```python
from build123d import *

# Parameters (mm, degrees)
F0_R     = 60
F1_DEPTH = 75
F2_R     = 45.05
F3_DEPTH = 300
F4_W     = 23.5
F4_H     = 7.8
F5_DEPTH = 78.9


with BuildPart() as f1:
    # F0 (on Front) → F1 (new body, symmetric)
    with BuildSketch(Plane.XZ):
        Circle(F0_R)
    extrude(amount=F1_DEPTH, both=True)

    # F2 (on face) → F3 (cut)
    with BuildSketch(Plane.XZ.offset(75)):
        Circle(F2_R)
    extrude(amount=-F3_DEPTH, mode=Mode.SUBTRACT)

    # F4 (on Right) → F5 (cut, symmetric)
    with BuildSketch(Plane.YZ):
        Rectangle(F4_W, F4_H)
    extrude(amount=F5_DEPTH, both=True, mode=Mode.SUBTRACT)


solid = f1.part
```
Geometry check sheet. Reference: the model listing, model coordinates, mm. A direction names the side the tool comes from. Round coordinates to 2 decimals unless told otherwise and drop trailing zeros. Order: outer loops, then holes, each group sorted by start corner. A loop starts at its lowest first (then second) coordinate and runs counter-clockwise, first axis right, second up. Notation, with made-up numbers: M 60.5,-23.75 L 79.5,-23.75 A23 ccw 79.5,-8.75 Z; hole C 69.5,78 d2. An arc over 180 degrees is marked long. Answer as CSV lines item,"result".
1) Gauge pin test, flat ends, axial feed: pin 1 Ø4.5 at (x, y) = (-49.5, 0) entering from +Z; pin 2 Ø7.5 at (x, y) = (52, -1) entering from -Z; pin 3 Ø12 at (x, y) = (-1, -22.5) entering from +Z. Record the tip position at first contact, or that the pin passes through.
Entries:
pin 1,"z = 36.98"
pin 2,"z = -35.66"
pin 3,"z = 60"
2) Sectioned sample at C-C on x = 0. Record the cut outline in (y, z).
Entries:
outline,"M -75,-60 L 75,-60 L 75,-45.05 L -75,-45.05 Z; M -75,45.05 L 75,45.05 L 75,60 L -75,60 Z"
3) Sectioned sample at D-D on y = -23. Record the cut outline in (x, z), and give its area (3 significant figures).
Entries:
outline,"C 0,0 d120; hole C 0,0 d90.1"
area,"4,930 mm2"
4) Mould release check, pull along X, two halves, no side actions. Record for faces 1 (the face through (52, 0, -3.9)), 2 (the face through (42.97, -1.05, 13.53)), 3 (the face through (55.425, -1.05, -22.98)): +X half, -X half, draft (parallel to the pull), parting line (faces both ways), or undercut.
Entries:
face 1,"draft"
face 2,"undercut"
face 3,"parting line"
5) Thickness scan on probe 1 along Z at (x, y) = (0, -0.5); probe 2 along Y at (x, z) = (-47, 1); probe 3 along Z at (x, y) = (34.5, -30). Record the ranges inside material, lowest first. Write a range as [from, to].
Entries:
probe 1,"[-60, -45.05], [45.05, 60]"
probe 2,"[-75, -11.75], [11.75, 75]"
probe 3,"[-49.09, -28.97], [28.97, 49.09]"
6) Sectioned sample at A-A on y = -7.5. Record the cut outline in (x, z), and give its area (3 significant figures).
Entries:
outline,"M -59.87,-3.9 A60 ccw 59.87,-3.9 L 44.88,-3.9 A45.05 cw -44.88,-3.9 Z; M -59.87,3.9 L -44.88,3.9 A45.05 cw 44.88,3.9 L 59.87,3.9 A60 ccw Z"
area,"4,700 mm2"
7) Sectioned sample at B-B on z = 0. Record the cut outline in (x, y).
Entries:
outline,"M -60,-75 L -45.05,-75 L -45.05,-11.75 L -60,-11.75 Z; M -60,11.75 L -45.05,11.75 L -45.05,75 L -60,75 Z; M 45.05,-75 L 60,-75 L 60,-11.75 L 45.05,-11.75 Z; M 45.05,11.75 L 60,11.75 L 60,75 L 45.05,75 Z"
8) Tool access check on faces 4 (the face through (-52, 0, 3.9)), 5 (the face through (9, 75, 45)). Record the directions out of +Z, -Z, +X, -X, +Y, -Y that give a thin tool (end or side, any length) a straight path to the whole face; none if there is none.
Entries:
face 4,"+X, -X"
face 5,"+Z, -Z, +X, -X, +Y"
